Could you check a few things on this model? Use its own coordinates, in mm. Face numbers are marked on the shaded views. Give positions to 0.01 mm unless a question says otherwise; leave off trailing zeros. Loops run counter-clockwise (first coordinate to the right, second up) from the corner with the lowest first, then second, coordinate; pieces in that order, holes last. Notation, with made-up numbers: (0.5, 54.5) - (22.5, 54.5) arc R12 ccw to (22.5, 59.5) - close; hole circle Ø8 at (-29.5, 67). An arc over 180 degrees is marked (long way). Write each question's results on one line, items separated by ' | '. Start each with the question number.
1) If I drill on probe 1 along Y at (x, z) = (-22.25, 4); probe 2 along X at (y, z) = (-4, 5.25); probe 3 along Y at (x, z) = (8, 2.5), over which ranges is the centre line in solid material (lowest first)? Write a range as [from, to].
2) I want a section at B-B, the plane y = -9. Write out the boundary of the cut face in (x, z).
3) I want a section at C-C, the plane x = -10.5. Write out the boundary of the cut face in (y, z), and give its area (3 significant figures).
4) I'm going to push a flat-ended pin straight in: pin 1 (2.5 mm diameter, centred on y = 16, z = 4, fed in from -X). Where does the tip first touch, or does it pass through?
5) If we mould it in two halves opening along X, with no side actions, what happens to the marked faces 1, 2 and 3? For each: +X half, -X half, draft (parallel to the pull), parting line (faces both ways), or undercut.
6) I want a section at A-A, the plane x = -24. Write out the boundary of the cut face in (y, z).
7) I want a section at D-D, the plane z = 4. Write out the boundary of the cut face in (x, y).
from build123d import *

# Parameters (mm, degrees)
SKETCH1_W           = 57
SKETCH1_H           = 42
BOSS_EXTRUDE1_DEPTH = 8
SKETCH2_R           = 17.5
SKETCH2_R_2         = 2
SKETCH2_R_3         = 1.5
CUT_EXTRUDE1_DEPTH  = 9
FILLET1_R           = 3
FILLET2_R           = 3
SKETCH3_R           = 2
CUT_EXTRUDE2_DEPTH  = 13


with BuildPart() as part:
    # Sketch1 → Boss-Extrude1 (new body)
    with BuildSketch(Plane.XY):
        Rectangle(SKETCH1_W, SKETCH1_H)
    extrude(amount=BOSS_EXTRUDE1_DEPTH)

    # Sketch2 → Cut-Extrude1 (cut, through all)
    with BuildSketch(Plane.XY.offset(8)):
        with Locations((8, 0)):
            Circle(SKETCH2_R)
        with Locations((25, 17.5)):
            Circle(SKETCH2_R_2)
        with Locations((-10.5, 17.5)):
            Circle(SKETCH2_R_2)
        with Locations((25, -17.5)):
            Circle(SKETCH2_R_2)
        with Locations((-10.5, -17.5)):
            Circle(SKETCH2_R_2)
        with Locations((-18.5, -11.5)):
            Circle(SKETCH2_R_3)
        with Locations((-24, -3.5)):
            Circle(SKETCH2_R_3)
    extrude(amount=-CUT_EXTRUDE1_DEPTH, mode=Mode.SUBTRACT)

    # Fillet1
    fillet1_edges = [part.edges().sort_by_distance(p)[0] for p in [
        (28.5, -21, 4),
    ]]
    fillet(fillet1_edges, radius=FILLET1_R)

    # Fillet2
    fillet2_edges = [part.edges().sort_by_distance(p)[0] for p in [
        (28.5, 21, 4),
    ]]
    fillet(fillet2_edges, radius=FILLET2_R)

    # Sketch3 → Cut-Extrude2 (cut)
    with BuildSketch(Plane.ZY.offset(28.5)):
        with Locations((4, 16)):
            Circle(SKETCH3_R)
        with Locations((4, -16)):
            Circle(SKETCH3_R)
    extrude(amount=-CUT_EXTRUDE2_DEPTH, mode=Mode.SUBTRACT)


solid = part.part
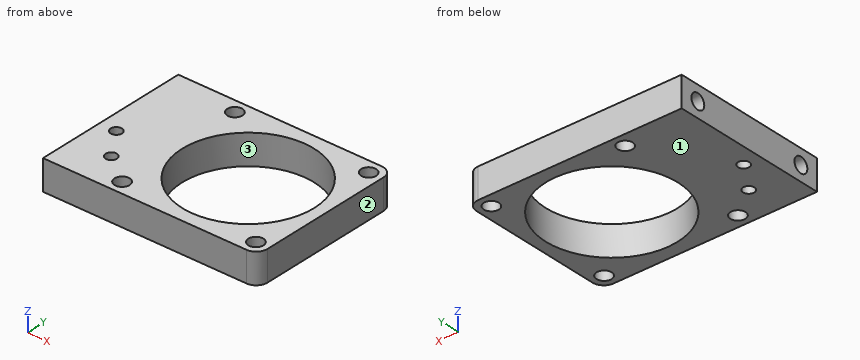
Answers:
1) probe 1: y = [-21, -18], [-14, 14], [18, 21] | probe 2: x = [-28.5, -25.41], [-22.59, -9.04], [25.04, 28.5] | probe 3: y = [-21, -17.5], [17.5, 21]
2) outline: (-28.5, 0) - (-7.01, 0) - (-7.01, 8) - (-28.5, 8) - close; (23.01, 0) - (28.5, 0) - (28.5, 8) - (23.01, 8) - close
3) outline: (-21, 0) - (-19.5, 0) - (-19.5, 8) - (-21, 8) - close; (-15.5, 0) - (15.5, 0) - (15.5, 8) - (-15.5, 8) - close; (19.5, 0) - (21, 0) - (21, 8) - (19.5, 8) - close | area: 272 mm2
4) pin 1: stops at x = -15.5
5) face 1: draft | face 2: +X half | face 3: undercut
6) outline: (-21, 0) - (-5, 0) - (-5, 8) - (-21, 8) - close; (-2, 0) - (21, 0) - (21, 8) - (-2, 8) - close; hole circle Ø4 at (-16, 4); hole circle Ø4 at (16, 4)
7) outline: (-28.5, -21) - (25.5, -21) arc R3 ccw to (28.5, -18) - (28.5, 18) arc R3 ccw to (25.5, 21) - (-28.5, 21) - (-28.5, 18) - (-15.5, 18) - (-15.5, 14) - (-28.5, 14) - (-28.5, -14) - (-15.5, -14) - (-15.5, -18) - (-28.5, -18) - close; hole circle Ø3 at (-24, -3.5); hole circle Ø3 at (-18.5, -11.5); hole circle Ø4 at (-10.5, -17.5); hole circle Ø4 at (-10.5, 17.5); hole circle Ø35 at (8, 0); hole circle Ø4 at (25, -17.5); hole circle Ø4 at (25, 17.5)
